```python
from build123d import *

# Parameters (mm, degrees)
SKETCH1_R           = 46
SKETCH1_R_2         = 2
BOSS_EXTRUDE1_DEPTH = 9
SKETCH2_R           = 23.5
CUT_EXTRUDE1_DEPTH  = 7
SKETCH3_R           = 20
CUT_EXTRUDE2_DEPTH  = 66.429351212
SKETCH4_R           = 3.5
CUT_EXTRUDE3_DEPTH  = 5
CUT_EXTRUDE4_DEPTH  = 5


with BuildPart() as part:
    # Sketch1 → Boss-Extrude1 (new body)
    with BuildSketch(Plane.XY):
        Circle(SKETCH1_R)
        with Locations((41.5, 0)):
            Circle(SKETCH1_R_2, mode=Mode.SUBTRACT)
        with Locations((20.75, -35.940054257)):
            Circle(SKETCH1_R_2, mode=Mode.SUBTRACT)
        with Locations((-20.75, -35.940054257)):
            Circle(SKETCH1_R_2, mode=Mode.SUBTRACT)
        with Locations((-41.5, 0)):
            Circle(SKETCH1_R_2, mode=Mode.SUBTRACT)
        with Locations((-20.75, 35.940054257)):
            Circle(SKETCH1_R_2, mode=Mode.SUBTRACT)
        with Locations((20.75, 35.940054257)):
            Circle(SKETCH1_R_2, mode=Mode.SUBTRACT)
    extrude(amount=BOSS_EXTRUDE1_DEPTH)

    # Sketch2 → Cut-Extrude1 (cut)
    with BuildSketch(Plane.XY.offset(9)):
        Circle(SKETCH2_R)
    extrude(amount=-CUT_EXTRUDE1_DEPTH, mode=Mode.SUBTRACT)

    # Sketch3 → Cut-Extrude2 (cut, through all)
    with BuildSketch(Plane.XY.offset(2)):
        Circle(SKETCH3_R)
    extrude(amount=-CUT_EXTRUDE2_DEPTH, mode=Mode.SUBTRACT)

    # Sketch4 → Cut-Extrude3 (cut)
    with BuildSketch(Plane(origin=(0, 0, 0), x_dir=(-1, 0, 0), z_dir=(0, 0, -1))):
        with Locations((-20.75, 35.940054257)):
            Circle(SKETCH4_R)
        with Locations((20.75, 35.940054257)):
            Circle(SKETCH4_R)
        with Locations((41.5, 0)):
            Circle(SKETCH4_R)
        with Locations((20.75, -35.940054257)):
            Circle(SKETCH4_R)
        with Locations((-20.75, -35.940054257)):
            Circle(SKETCH4_R)
        with Locations((-41.5, 0)):
            Circle(SKETCH4_R)
    extrude(amount=-CUT_EXTRUDE3_DEPTH, mode=Mode.SUBTRACT)

    # Sketch5 → Cut-Extrude4 (cut)
    with BuildSketch(Plane(origin=(0, 0, 0), x_dir=(-1, 0, 0), z_dir=(0, 0, -1))):
        with BuildLine():
            Line((-41.5, 3.5), (-45.866654554, 3.5))
            ThreePointArc((-45.866654554, 3.5), (-46, 0), (-45.866654554, -3.5))
            Line((-45.866654554, -3.5), (-41.5, -3.5))
            ThreePointArc((-41.5, -3.5), (-45, 0), (-41.5, 3.5))
        make_face()
        with BuildLine():
            ThreePointArc((-23.781088913, 34.190054257), (-22.5, 38.97114317), (-17.718911087, 37.690054257))
            Line((-17.718911087, 37.690054257), (-19.902238364, 41.471688031))
            ThreePointArc((-19.902238364, 41.471688031), (-23, 39.837168574), (-25.96441619, 37.971688031))
            Line((-25.96441619, 37.971688031), (-23.781088913, 34.190054257))
        make_face()
        with BuildLine():
            ThreePointArc((25.96441619, 37.971688031), (23, 39.837168574), (19.902238364, 41.471688031))
            Line((19.902238364, 41.471688031), (17.718911087, 37.690054257))
            ThreePointArc((17.718911087, 37.690054257), (21.655866658, 39.320794649), (24.25, 35.940054257))
            ThreePointArc((24.25, 35.940054257), (24.130740392, 35.034187599), (23.781088913, 34.190054257))
            Line((23.781088913, 34.190054257), (25.96441619, 37.971688031))
        make_face()
        with BuildLine():
            ThreePointArc((46, 0), (45.96665155, 1.751269611), (45.866654554, 3.5))
            Line((45.866654554, 3.5), (41.5, 3.5))
            ThreePointArc((41.5, 3.5), (43.974873734, 2.474873734), (45, 0))
            ThreePointArc((45, 0), (43.974873734, -2.474873734), (41.5, -3.5))
            Line((41.5, -3.5), (45.866654554, -3.5))
            ThreePointArc((45.866654554, -3.5), (45.96665155, -1.751269611), (46, 0))
        make_face()
        with BuildLine():
            Line((17.718911087, -37.690054257), (19.902238364, -41.471688031))
            ThreePointArc((19.902238364, -41.471688031), (23, -39.837168574), (25.96441619, -37.971688031))
            Line((25.96441619, -37.971688031), (23.781088913, -34.190054257))
            ThreePointArc((23.781088913, -34.190054257), (24.130740392, -35.034187599), (24.25, -35.940054257))
            ThreePointArc((24.25, -35.940054257), (21.655866658, -39.320794649), (17.718911087, -37.690054257))
        make_face()
        with BuildLine():
            Line((-23.781088913, -34.190054257), (-25.96441619, -37.971688031))
            ThreePointArc((-25.96441619, -37.971688031), (-23, -39.837168574), (-19.902238364, -41.471688031))
            Line((-19.902238364, -41.471688031), (-17.718911087, -37.690054257))
            ThreePointArc((-17.718911087, -37.690054257), (-22.5, -38.97114317), (-23.781088913, -34.190054257))
        make_face()
    extrude(amount=-CUT_EXTRUDE4_DEPTH, mode=Mode.SUBTRACT)


solid = part.part
```
Check sheet for the modelled part. Datum: model origin and axes. Units: mm. A direction names the side the tool comes from. Round coordinates to 2 decimals unless told otherwise and drop trailing zeros. Order: outer loops, then holes, each group sorted by start corner. A loop starts at its lowest first (then second) coordinate and runs counter-clockwise, first axis right, second up. Notation, with made-up numbers: (75, 68.25) -> (124, 68.25) arc R19 cw to (124, 84.25) -> close; hole circle Ø1 at (43.5, 46). An arc over 180 degrees is marked (long way). One line per item, written item: value. Start each with the question number.
Q1. Cross-section at B-B (x = 9). Record the boundary of the cut face in (y, z).
Q2. Gauge pin test, flat ends, axial feed: pin 1 Ø5 at (x, z) = (-43, 3) entering from +Y; pin 2 Ø5 at (x, z) = (-43.5, 3.5) entering from -Y; pin 3 Ø3 at (y, z) = (-13, 5.5) entering from +X. Record the tip position at first contact, or that the pin passes through.
Q3. Thickness scan on line 1 (X direction, y = -34.5, z = 1.25); line 2 (Y direction, x = 42, z = 3); line 3 (Y direction, x = 20.75, z = 7.5). Record the ranges inside material, lowest first.
Q4. Cross-section at A-A (y = 0). Record the boundary of the cut face in (x, z), and give its area (3 significant figures).
Q5. Mould release check, pull along Y, two halves, no side actions. Record for faces 1 (the face through (-1, 21, 0)), 2 (the face through (24.857, -36.054, 2.465)), 3 (the face through (-22, 38, 5)): pulls with the +Y half, pulls with the -Y half, needs draft (parallel to the pull), parting line crosses it, or undercut.
Q6. Cross-section at C-C (z = 7.75). Record the boundary of the cut face in (x, y).
Q7. Cross-section at D-D (x = -1). Record the boundary of the cut face in (y, z).
Q8. Set-up check for faces 4 (the face through (38, 0, 2)), 5 (the face through (-19.07, -32.87, 2.46)), 6 (the face through (24.89, 36.11, 2.46)), 7 (the face through (-44, 3.5, 2)), 8 (the face through (7, 19, 2)): record each of +Z, -Z, +X, -X, +Y, -Y from which the full face is reachable in a straight line by a thin tool's end or side.
Completed:
1. outline: (-45.11, 0) -> (-17.86, 0) -> (-17.86, 2) -> (-21.71, 2) -> (-21.71, 9) -> (-45.11, 9) -> close; (17.86, 0) -> (45.11, 0) -> (45.11, 9) -> (21.71, 9) -> (21.71, 2) -> (17.86, 2) -> close
2. pin 1: stops at y = 21.81
2. pin 2: stops at y = -20.86
2. pin 3: stops at x = 44.54
3. line 1: x = -30.43 to -23.96, -17.56 to 17.56, 23.96 to 30.43
3. line 2: y = -18.76 to -3.5, 3.5 to 18.76
3. line 3: y = -41.05 to -37.94, -33.94 to -11.03, 11.03 to 33.94, 37.94 to 41.05
4. outline: (-46, 5) -> (-43.5, 5) -> (-43.5, 9) -> (-46, 9) -> close; (-39.5, 5) -> (-38, 5) -> (-38, 0) -> (-20, 0) -> (-20, 2) -> (-23.5, 2) -> (-23.5, 9) -> (-39.5, 9) -> close; (20, 0) -> (38, 0) -> (38, 5) -> (39.5, 5) -> (39.5, 9) -> (23.5, 9) -> (23.5, 2) -> (20, 2) -> close; (43.5, 5) -> (46, 5) -> (46, 9) -> (43.5, 9) -> close
4. area: 307 mm²
5. face 1: needs draft
5. face 2: pulls with the -Y half
5. face 3: undercut
6. outline: circle Ø92 at (0, 0); hole circle Ø4 at (-41.5, 0); hole circle Ø47 at (0, 0); hole circle Ø4 at (-20.75, -35.94); hole circle Ø4 at (-20.75, 35.94); hole circle Ø4 at (20.75, -35.94); hole circle Ø4 at (20.75, 35.94); hole circle Ø4 at (41.5, 0)
7. outline: (-45.99, 0) -> (-19.97, 0) -> (-19.97, 2) -> (-23.48, 2) -> (-23.48, 9) -> (-45.99, 9) -> close; (19.97, 0) -> (45.99, 0) -> (45.99, 9) -> (23.48, 9) -> (23.48, 2) -> (19.97, 2) -> close
8. face 4: -Z, +X
8. face 5: -Z
8. face 6: -Z, +Y
8. face 7: -Z, -X
8. face 8: +Z
